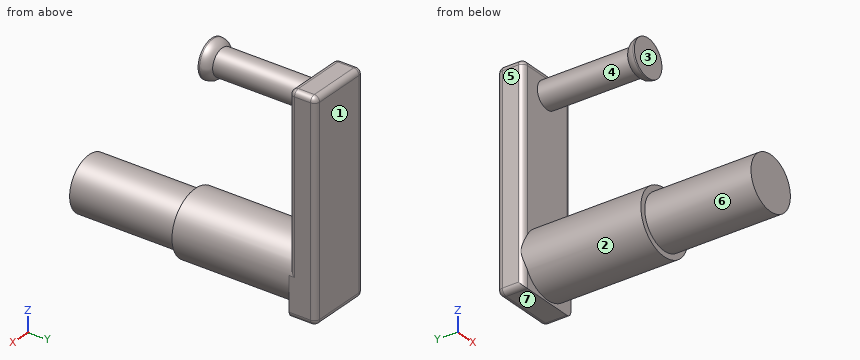
Autodesk Inventor part; units mm, degrees
ref_plane "YZ Plane" through (0, 0, 0) normal (1, 0, 0) x (0, 1, 0)
ref_plane "XZ Plane" through (0, 0, 0) normal (0, 1, 0) x (-1, 0, 0)
ref_plane "XY Plane" through (0, 0, 0) normal (0, 0, 1) x (1, 0, 0)
sketch "Sketch1" plane through (0, 0, 0) normal (0, 1, 0) x (-1, 0, 0)
  circle A0 centre (0, 0) radius 5
  circle A1 centre (0, 0) radius 6
  dimension "d0" = 10
  dimension "d1" = 12
extrude "Extrusion1" add sketch "Sketch1" against normal blind 20 contours A0
extrude "Extrusion2" add sketch "Sketch1" along normal blind 22 contours A0 | A1
sketch "Sketch2" plane through (0, 22, 0) normal (0, 1, 0) x (1, 0, 0)
  line L0 (-6.0998, -33.6689) -> (5.9002, -33.6689)
  line L1 (5.9002, -33.6689) -> (5.9002, 6.3311)
  line L2 (5.9002, 6.3311) -> (-6.0998, 6.3311)
  line L3 (-6.0998, 6.3311) -> (-6.0998, -33.6689)
  circle A0 centre (-0.0998, -29.7677) radius 2.5
  point P0 (0, 0)
  dimension "d8" = 12
  dimension "d9" = 40
  dimension "d15" = 5
extrude "Extrusion3" add sketch "Sketch2" along normal blind 5 contours L3 L2 L1 L0 | A0
fillet "Fillet1" radius 1 11 edges at (5.9002, 27, 13.6689) (5.9002, 22, 17.3793) (5.9002, 24.5, -6.3311) (-0.0998, 27, -6.3311) (-6.0998, 27, 13.6689) (-0.0998, 27, 33.6689) (-6.0998, 24.5, 33.6689) (-6.0998, 22, 13.6689) (-6.0998, 24.5, -6.3311) (-0.0998, 22, 33.6689) (5.9002, 24.5, 33.6689)
thread "Thread1"
extrude "Extrusion4" add sketch "Sketch2" against normal blind 17 contours A0
sketch "Sketch3" plane through (-0.0998, 5, 29.7677) normal (0, -1, 0) x (1, 0, 0)
  circle A0 centre (0, 0) radius 3.5
  point P0 (0.0998, -29.7677)
  dimension "d18" = 7
extrude "Extrusion5" add sketch "Sketch3" along normal blind 2
fillet "Fillet2" radius 2 1 edges at (-3.5998, 5, 29.7677)
sketch "Sketch4" plane through (-0.0998, 3, 29.7677) normal (0, -1, 0) x (1, 0, 0)
  point P0 (0.0998, -29.7677)
properties part number "clamp" material "Steel, Carbon"
Model file for the job. Use its own axes, mm. Face numbers are marked on the shaded views. A direction names the side the tool comes from. Give positions to 0.01 mm unless a question says otherwise; leave off trailing zeros. Order: outer loops, then holes, each group sorted by start corner. A loop starts at its lowest first (then second) coordinate and runs counter-clockwise, first axis right, second up. Notation, with made-up numbers: (-8.5, -39.5) - (39.5, -39.5) arc R14 ccw to (39.5, -30.5) - close; hole circle Ø9 at (75.5, 87.5). An arc over 180 degrees is marked (long way). Return JSON: item names as keys, results as strings.
1) Cut at C-C, the plane y = 17. Give the cut face in (x, z), plus the area to 3 significant figures.
Geometry says:
{"outline": "circle Ø12 at (0, 0); circle Ø5 at (-0.1, 29.77)", "area": "133 mm²"}
2) Cut at D-D, the plane z = 0. Give the cut face in (x, y), plus the area to 4 significant figures.
Geometry says:
{"outline": "(-6.1, 23) arc R1 ccw to (-6, 22.56) - (-6, 0) - (-5, 0) - (-5, -20) - (5, -20) - (5, 0) - (6, 0) - (6, 22) - (5.9, 22) - (5.9, 26) arc R1 ccw to (4.9, 27) - (-5.1, 27) arc R1 ccw to (-6.1, 26) - close", "area": "523.5 mm²"}
3) Cut at B-B, the plane y = 1. Give the cut face in (x, z), plus the area to 3 significant figures.
Geometry says:
{"outline": "circle Ø12 at (0, 0)", "area": "113 mm²"}
4) 3-axis set-ups, long thin cutter, end or side, ignore diameter. For the marked faces 1, 2 and 3: which of +Z, -Z, +X, -X, +Y, -Y reach the whole face in a straight line?
Geometry says:
{"face 1": "+Z, -Z, +X, -X, +Y", "face 2": "-Y", "face 3": "+Z, +X, -X, -Y"}
5) Probe line 1 (Z direction, x = 0.25, y = -4); line 2 (Y direction, x = -4.5, z = 8); line 3 (Z direction, x = 0.5, y = 7). List the from-to ranges inside material, lowest first. Write a range as from..to.
Geometry says:
{"line 1": "-4.99..4.99", "line 2": "22..27", "line 3": "-5.98..5.98, 27.34..32.19"}
6) Flat gauge pins, fed straight in: P1, Ø6, axis at x = -2, z = 11, coming from the -Y side; P2, Ø2, axis at x = 1.5, z = 31.5, coming from the -Y side; P3, Ø1.5, axis at x = 2, y = -2, coming from the +Z side. Where does each tip first touch, or does it go through?
Geometry says:
{"P1": "y = 22", "P2": "y = 3", "P3": "z = 4.84"}
7) Pull direction Z, two halves, no side cores. Call the marked faces 4, 5, 6 and 7: pulls with the +Z half, pulls with the -Z half, needs draft (parallel to the pull), parting line crosses it, or undercut.
Geometry says:
{"face 4": "undercut", "face 5": "needs draft", "face 6": "parting line crosses it", "face 7": "pulls with the -Z half"}
8) Cut at A-A, the plane z = 17. Give the cut face in (x, y).
Geometry says:
{"outline": "(-6.1, 23) arc R1 ccw to (-5.1, 22) - (4.9, 22) arc R1 ccw to (5.9, 23) - (5.9, 26) arc R1 ccw to (4.9, 27) - (-5.1, 27) arc R1 ccw to (-6.1, 26) - close"}
